Model file for the job. Use its own axes, mm. Face numbers are marked on the shaded views. A direction names the side the tool comes from. Coordinates: 2 decimals unless noted, no trailing zeros. Write each loop counter-clockwise with the first axis right and the second up, starting at its lowest first coordinate (ties: lowest second). Pieces come first, ordered by that corner, then holes. Notation, with made-up numbers: (13, -34.5) -> (56, -34.5) arc R23 ccw to (56, -23.5) -> close; hole circle Ø4 at (-37, -11). An arc over 180 degrees is marked (long way). Answer as a JSON object with one key per item and string values. Group by question number.
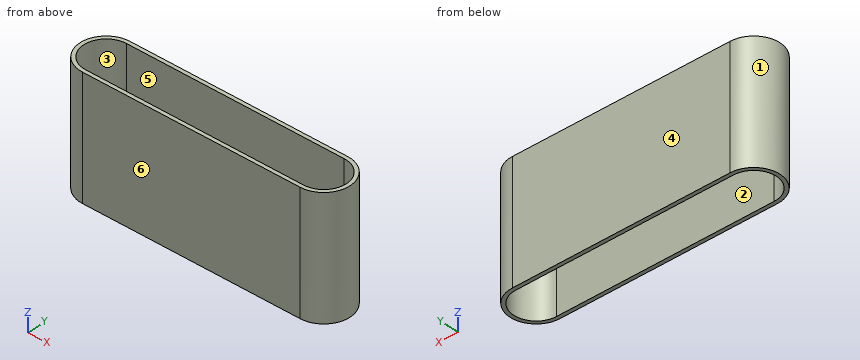
Autodesk Inventor part; units mm, degrees
ref_plane "YZ Plane" through (0, 0, 0) normal (1, 0, 0) x (0, 1, 0)
ref_plane "XZ Plane" through (0, 0, 0) normal (0, 1, 0) x (-1, 0, 0)
ref_plane "XY Plane" through (0, 0, 0) normal (0, 0, 1) x (1, 0, 0)
sketch "Sketch1" plane through (0, 0, 0) normal (0, 0, 1) x (1, 0, 0)
  line L0 (0, 0) -> (-222.25, 0) construction
  line L1 (-19.05, 19.05) -> (-203.2, 19.05)
  line L2 (-203.2, -19.05) -> (-19.05, -19.05)
  arc A0 (-19.05, -19.05) -> (-19.05, 19.05) centre (-19.05, 0) ccw
  arc A1 (-203.2, 19.05) -> (-203.2, -19.05) centre (-203.2, 0) ccw
  line L3 (0, 0) -> (222.25, 0) construction
  line L4 (-203.2, 22.225) -> (-19.05, 22.225)
  arc A2 (-19.05, -22.225) -> (-19.05, 22.225) centre (-19.05, 0) ccw
  line L5 (-19.05, -22.225) -> (-203.2, -22.225)
  arc A3 (-203.2, 22.225) -> (-203.2, -22.225) centre (-203.2, 0) ccw
  point P0 (-111.125, 0)
  dimension "d0" = 222.25
  dimension "d1" = 180
  dimension "d2" = 38.1
  dimension "d3" = 3.175
extrude "Extrusion1" add sketch "Sketch1" along normal blind 101.6
properties part number "Shooting_Belt_2"
(1) Cut at A-A on y = 0. List the corners of the cut face in (x, z) (3 decimals), plus the area to 3 significant figures.
(2) 3-axis set-ups, long thin cutter, end or side, ignore diameter. For the marked faces 1 and 2: which of +Z, -Z, +X, -X, +Y, -Y reach the whole face in a straight line?
(3) Cut at B-B on x = -84. List the corners of the cut face in (y, z) (3 decimals).
(4) Wall check: probe 1 along Y at (x, z) = (-144, 58.5) (3 decimals); probe 2 along X at (y, z) = (1, 38.5); probe 3 along X at (y, z) = (-6, 58.5). Give the ranges that are in metal, low to high.
(5) Pin check, flat tips, straight feed: pin 1 (1 mm diameter, centred on y = -16, z = 70, fed in from -X); pin 2 (8 mm diameter, centred on x = -79.5, y = -17.5, fed in from +Z); pin 3 (1 mm diameter, centred on y = 17.5, z = 61, fed in from +X); pin 4 (3 mm diameter, centred on y = -9.5, z = 55.5, fed in from +X). Stop position of each tip, or through.
(6) Pull direction Y, two halves, no side cores. Call the marked faces 3, 4, 5 and 6: released by +Y, released by -Y, zero draft, split by the parting line, or undercut.
(7) Cut at C-C on z = 12.5. List the corners of the cut face in (x, y) (3 decimals).
Results found:
{
 "1": {"outline": "(-225.425, 0) -> (-222.25, 0) -> (-222.25, 101.6) -> (-225.425, 101.6) -> close; (0, 0) -> (3.175, 0) -> (3.175, 101.6) -> (0, 101.6) -> close", "area": "645 mm²"},
 "2": {"face 1": "+Z, -Z, -X", "face 2": "+Z, -Z"},
 "3": {"outline": "(-22.225, 0) -> (-19.05, 0) -> (-19.05, 101.6) -> (-22.225, 101.6) -> close; (19.05, 0) -> (22.225, 0) -> (22.225, 101.6) -> (19.05, 101.6) -> close"},
 "4": {"probe 1": "y = -22.225 to -19.05, 19.05 to 22.225", "probe 2": "x = -225.4 to -222.22, -0.03 to 3.15", "probe 3": "x = -224.6 to -221.28, -0.97 to 2.35"},
 "5": {"pin 1": "stops at x = -219.13", "pin 2": "stops at z = 101.6", "pin 3": "stops at x = -4.73", "pin 4": "stops at x = 1.69"},
 "6": {"face 3": "undercut", "face 4": "released by +Y", "face 5": "undercut", "face 6": "released by -Y"},
 "7": {"outline": "(-203.2, -22.225) -> (-19.05, -22.225) arc R22.225 ccw to (-19.05, 22.225) -> (-203.2, 22.225) arc R22.225 ccw to start; hole (-203.2, -19.05) -> (-19.05, -19.05) arc R19.05 ccw to (-19.05, 19.05) -> (-203.2, 19.05) arc R19.05 ccw to start"}
}
